Verification items for the finished model (mm, model axes). A direction names the side the tool comes from. Give positions to 0.01 mm unless a question says otherwise; leave off trailing zeros. Order: outer loops, then holes, each group sorted by start corner. A loop starts at its lowest first (then second) coordinate and runs counter-clockwise, first axis right, second up.
from build123d import *

# Parameters (mm, degrees)
F0_W     = 25.4
F0_H     = 12.7
F1_DEPTH = 330.2
F2_W     = 38.1
F2_H     = 12.7
F3_DEPTH = 457.201
F4_W     = 50.8
F4_H     = 12.7
F5_DEPTH = 584.2


with BuildPart() as f1:
    # F0 (on Right) → F1 (new body, symmetric)
    with BuildSketch(Plane.YZ):
        with Locations((-215.9, -6.35)):
            Rectangle(F0_W, F0_H)
        Polygon((-228.6, 15.08125), (-228.6, 0), (-203.2, 0), (203.2, 0), (228.6, 0), (228.6, 15.08125), align=None)
        with Locations((215.9, -6.35)):
            Rectangle(F0_W, F0_H)
    extrude(amount=F1_DEPTH, both=True)

    # F2 (on face) → F3 (cut, through all)
    with BuildSketch(Plane.XZ.offset(228.6)):
        with Locations((-311.15, -6.35)):
            Rectangle(F2_W, F2_H)
        with Locations((311.15, -6.35)):
            Rectangle(F2_W, F2_H)
    extrude(amount=-F3_DEPTH, mode=Mode.SUBTRACT)

    # F4 (on face) → F5 (join, through all)
    with BuildSketch(Plane(origin=(-292.1, 0, 0), x_dir=(0, -1, 0), z_dir=(-1, 0, 0))):
        with Locations((0, -6.35)):
            Rectangle(F4_W, F4_H)
    extrude(amount=-F5_DEPTH)


solid = f1.part
(1) Section check A-A, the plane z = -7. Enter the section's corners in (x, y).
Solved:
outline: (-292.1, -228.6) - (292.1, -228.6) - (292.1, -203.2) - (-292.1, -203.2) - close; (-292.1, -25.4) - (292.1, -25.4) - (292.1, 25.4) - (-292.1, 25.4) - close; (-292.1, 203.2) - (292.1, 203.2) - (292.1, 228.6) - (-292.1, 228.6) - close
(2) Section check C-C, the plane y = -84. Enter the section's corners in (x, z).
Solved:
outline: (-330.2, 0) - (330.2, 0) - (330.2, 15.08) - (-330.2, 15.08) - close
(3) Section check B-B, the plane x = -135.5. Enter the section's corners in (y, z), then the cut area to 3 significant figures.
Solved:
outline: (-228.6, -12.7) - (-203.2, -12.7) - (-203.2, 0) - (-25.4, 0) - (-25.4, -12.7) - (25.4, -12.7) - (25.4, 0) - (203.2, 0) - (203.2, -12.7) - (228.6, -12.7) - (228.6, 15.08) - (-228.6, 15.08) - close
area: 8,190 mm2
(4) Set-up check for faces 1 (the flat face through (330.2, -3, 8)), 2 (the flat face through (4, 216, -12.7)), 3 (the flat face through (-292.1, -216, -6)), 4 (the flat face through (4, 203.2, -6)), 5 (the flat face through (292.1, 0, -6)): record each of +Z, -Z, +X, -X, +Y, -Y from which the full face is reachable in a straight line by a thin tool's end or side.
Solved:
face 1: +Z, -Z, +X, +Y, -Y
face 2: -Z, +X, -X, +Y, -Y
face 3: -Z, -X, +Y, -Y
face 4: -Z, +X, -X
face 5: -Z, +X, +Y, -Y
(5) Go/stop test with flat-tipped pins: pin 1 (3 mm diameter, centred on x = -210.5, y = 78, fed in from -Z); pin 2 (6.5 mm diameter, centred on y = 12, z = -5, fed in from -X); pin 3 (4 mm diameter, centred on y = -11, z = -3.5, fed in from +X). Record where each tip stops, or that it passes through.
Solved:
pin 1: stops at z = 0
pin 2: stops at x = -292.1
pin 3: stops at x = 292.1
(6) Release check for a two-part mould opening along Y. For faces 6 (the flat face through (-4, -25.4, -6)), 7 (the flat face through (4, -216, -12.7)), 8 (the flat face through (5, -228.6, 1)) record: pulls with the +Y half, pulls with the -Y half, needs draft (parallel to the pull), parting line crosses it, or undercut.
Solved:
face 6: undercut
face 7: needs draft
face 8: pulls with the -Y half
(7) Scan lines: line 1 (Y direction, x = 180, z = -3.25); line 2 (Z direction, x = -34, y = -151.5). Record each from-to range of solid material in increasing order.
Solved:
line 1: y = -228.6 to -203.2, -25.4 to 25.4, 203.2 to 228.6
line 2: z = 0 to 15.08
